from build123d import *

# Parameters (mm, degrees)
EXTRUDE_THIN1_DEPTH = 37.34
SKETCH2_R           = 1.83
CUT_EXTRUDE1_DEPTH  = 11.52
SKETCH3_W           = 44.45
SKETCH3_H           = 2.5
CUT_EXTRUDE2_DEPTH  = 8


with BuildPart() as part:
    # Sketch1 → Extrude-Thin1 (new body)
    with BuildSketch(Plane(origin=(0, 0, 0), x_dir=(1, 0, 0), z_dir=(0, 1, 0))):
        with BuildLine():
            Line((-22.225, 9.52), (-9.14, 9.52))
            ThreePointArc((-9.14, 9.52), (-8.963223305, 9.446776695), (-8.89, 9.27))
            Line((-8.89, 9.27), (-8.89, 1.25))
            ThreePointArc((-8.89, 1.25), (-8.523883476, 0.366116524), (-7.64, 0))
            Line((-7.64, 0), (7.64, 0))
            ThreePointArc((7.64, 0), (8.523883476, 0.366116524), (8.89, 1.25))
            Line((8.89, 1.25), (8.89, 9.27))
            ThreePointArc((8.89, 9.27), (8.963223305, 9.446776695), (9.14, 9.52))
            Line((9.14, 9.52), (22.225, 9.52))
            Line((22.225, 9.52), (22.225, 10.52))
            Line((22.225, 10.52), (9.14, 10.52))
            ThreePointArc((9.14, 10.52), (8.256116524, 10.153883476), (7.89, 9.27))
            Line((7.89, 9.27), (7.89, 1.25))
            ThreePointArc((7.89, 1.25), (7.816776695, 1.073223305), (7.64, 1))
            Line((7.64, 1), (-7.64, 1))
            ThreePointArc((-7.64, 1), (-7.816776695, 1.073223305), (-7.89, 1.25))
            Line((-7.89, 1.25), (-7.89, 9.27))
            ThreePointArc((-7.89, 9.27), (-8.256116524, 10.153883476), (-9.14, 10.52))
            Line((-9.14, 10.52), (-22.225, 10.52))
            Line((-22.225, 10.52), (-22.225, 9.52))
        make_face()
    extrude(amount=EXTRUDE_THIN1_DEPTH)

    # Sketch2 → Cut-Extrude1 (cut, through all)
    with BuildSketch(Plane.XY):
        with Locations((0, 13.59)):
            Circle(SKETCH2_R)
        with Locations((0, 23.75)):
            Circle(SKETCH2_R)
    extrude(amount=-CUT_EXTRUDE1_DEPTH, mode=Mode.SUBTRACT)

    # Sketch3 → Cut-Extrude2 (cut)
    with BuildSketch(Plane(origin=(0, 0, -10.52), x_dir=(-1, 0, 0), z_dir=(0, 0, -1))):
        with Locations((0, 31.95)):
            Rectangle(SKETCH3_W, SKETCH3_H)
        with Locations((0, 25.31)):
            Rectangle(SKETCH3_W, SKETCH3_H)
        with Locations((0, 18.67)):
            Rectangle(SKETCH3_W, SKETCH3_H)
        with Locations((0, 12.03)):
            Rectangle(SKETCH3_W, SKETCH3_H)
        with Locations((0, 5.39)):
            Rectangle(SKETCH3_W, SKETCH3_H)
    extrude(amount=-CUT_EXTRUDE2_DEPTH, mode=Mode.SUBTRACT)


solid = part.part
Geometry: final body of the model. Coordinates: model frame, mm. A direction names the side the tool comes from. Coordinates: 2 decimals unless noted, no trailing zeros. Write each loop counter-clockwise with the first axis right and the second up, starting at its lowest first coordinate (ties: lowest second). Pieces come first, ordered by that corner, then holes. Notation, with made-up numbers: (48.25, 17.25) - (64.25, 17.25) arc R12 ccw to (64.25, 39.25) - close; hole circle Ø6 at (2.25, 74). An arc over 180 degrees is marked (long way). Return JSON: item names as keys, results as strings.
Item 1: Section query A-A (x = 0). Output: boundary loops of the cut face in (y, z), and give its area (3 significant figures).
Completed:
{"outline": "(0, -1) - (11.76, -1) - (11.76, 0) - (0, 0) - close; (15.42, -1) - (21.92, -1) - (21.92, 0) - (15.42, 0) - close; (25.58, -1) - (37.34, -1) - (37.34, 0) - (25.58, 0) - close", "area": "30.0 mm2"}
Item 2: Line query: L1, parallel to Y at x = 0, z = -0.6; L2, parallel to X at y = 3, z = -1.75; L3, parallel to Z at x = 14.5, y = 3.5. Output: solid intervals per line, ascending.
Completed:
{"L1": "y = 0 to 11.76, 15.42 to 21.92, 25.58 to 37.34", "L2": "x = -8.89 to -7.89, 7.89 to 8.89", "L3": "z = -10.52 to -9.52"}
Item 3: Section query C-C (y = 20.5). Output: boundary loops of the cut face in (x, z) (3 decimals).
Completed:
{"outline": "(-22.225, -10.52) - (-9.14, -10.52) arc R1.25 ccw to (-7.89, -9.27) - (-7.89, -1.25) arc R0.25 cw to (-7.64, -1) - (7.64, -1) arc R0.25 cw to (7.89, -1.25) - (7.89, -9.27) arc R1.25 ccw to (9.14, -10.52) - (22.225, -10.52) - (22.225, -9.52) - (9.14, -9.52) arc R0.25 cw to (8.89, -9.27) - (8.89, -1.25) arc R1.25 ccw to (7.64, 0) - (-7.64, 0) arc R1.25 ccw to (-8.89, -1.25) - (-8.89, -9.27) arc R0.25 cw to (-9.14, -9.52) - (-22.225, -9.52) - close"}
Item 4: Pull-direction query (X, two-part tool) for faces 1 (the face through (-8.246, 35.241, -10.144)), 2 (the face through (8.89, 18, -2)), 3 (the face through (-22.225, 2, -10)), 4 (the face through (-16, 2, -10.52)); classes: +X half, -X half, draft (parallel to the pull), parting line (faces both ways), or undercut.
Completed:
{"face 1": "undercut", "face 2": "+X half", "face 3": "-X half", "face 4": "draft"}
Item 5: Section query D-D (z = -4.5). Count the separate pieces of the cut face and the enclosed holes in it, and give its area (3 significant figures).
Completed:
{"separate pieces": "12", "enclosed holes": "0", "area": "49.7 mm2"}
Item 6: Section query B-B (x = 17). Output: boundary loops of the cut face in (y, z).
Completed:
{"outline": "(0, -10.52) - (4.14, -10.52) - (4.14, -9.52) - (0, -9.52) - close; (6.64, -10.52) - (10.78, -10.52) - (10.78, -9.52) - (6.64, -9.52) - close; (13.28, -10.52) - (17.42, -10.52) - (17.42, -9.52) - (13.28, -9.52) - close; (19.92, -10.52) - (24.06, -10.52) - (24.06, -9.52) - (19.92, -9.52) - close; (26.56, -10.52) - (30.7, -10.52) - (30.7, -9.52) - (26.56, -9.52) - close; (33.2, -10.52) - (37.34, -10.52) - (37.34, -9.52) - (33.2, -9.52) - close"}
Item 7: Reachability of faces 5 (the face through (22.225, 22, -10)), 6 (the face through (-12, 4.14, -10)), 7 (the face through (-16, 29, -9.52)), 8 (the face through (-8.246, 15.321, -10.144)) from +Z, -Z, +X, -X, +Y, -Y: full face, straight path, thin tool, end or side. Return the list, or none.
Completed:
{"face 5": "+Z, -Z, +X, +Y, -Y", "face 6": "-Z, +X, -X", "face 7": "+Z, -X, +Y, -Y", "face 8": "-Z, +Y, -Y"}
Item 8: Pin query (flat end, axial travel): pin 1 Ø0.5 at (x, y) = (8.5, 5) entering from -Z; pin 2 Ø6 at (y, z) = (12, -6) entering from +X; pin 3 Ø1 at (y, z) = (32.5, -5.5) entering from -X; pin 4 Ø10 at (x, y) = (-0.5, 14) entering from -Z. Return the tip coordinate at first contact, or that it passes through.
Completed:
{"pin 1": "stops at z = -2.52", "pin 2": "stops at x = 8.89", "pin 3": "passes through", "pin 4": "stops at z = -1"}
